Geometry check sheet. Reference: the model listing, model coordinates, mm. A direction names the side the tool comes from. Give positions to 0.01 mm unless a question says otherwise; leave off trailing zeros. Write each loop counter-clockwise with the first axis right and the second up, starting at its lowest first coordinate (ties: lowest second). Pieces come first, ordered by that corner, then holes.
(1) Cross-section at D-D (x = -6). Record the boundary of the cut face in (y, z).
(2) Mould release check, pull along Y, two halves, no side actions. Record for faces 4 (the flat face through (-10.447, 4.997, 0.071)), 5 (the flat face through (-19, -9.906, 0)), 6 (the flat face through (0, 20.32, 0)), 7 (the flat face through (-19, 0, 2.286)): +Y half, -Y half, draft (parallel to the pull), parting line (faces both ways), or undercut.
(3) Cross-section at C-C (y = 12). Record the boundary of the cut face in (x, z).
(4) Tool access check on faces 1 (the flat face through (-1, 11.232, 0)), 2 (the flat face through (-19, 9.906, 0)), 3 (the flat face through (-10.16, -17, 0)). Record the directions out of +Z, -Z, +X, -X, +Y, -Y that give a thin tool (end or side, any length) a straight path to the whole face; none if there is none.
(5) Cross-section at B-B (y = -8.5). Record the boundary of the cut face in (x, z), and give its area (3 significant figures).
(6) Depth check by flat-ended pin: P1, Ø1.3, axis at x = -18.5, z = -0.5, coming from the -Y side; P2, Ø1.3, axis at x = -19.5, z = 1, coming from the +Y side; P3, Ø12, axis at x = 0, y = 4, coming from the +Z side; P4, Ø1.3, axis at y = 19, z = 0, coming from the -X side. Enter the tip coordinate at first touch or a pass-through.
(7) Thickness scan on line 1 along X through (y, z) = (3.5, 1.25); line 2 along X through (y, z) = (-4.5, 0.5); line 3 along X through (y, z) = (8, -0.5). Record the ranges inside material, lowest first.
(8) Cross-section at A-A (x = 8). Record the boundary of the cut face in (y, z), and give its area (3 significant figures).
```python
from build123d import *

# Parameters (mm, degrees)
F0_W     = 35.56
F0_H     = 35.56
F1_DEPTH = 5.08
F2_W     = 19.812
F2_H     = 4.572
F3_DEPTH = 2.54
F4_W     = 19.812
F4_H     = 4.572
F5_DEPTH = 2.54
F6_W     = 20.32
F6_H     = 5.08
F7_DEPTH = 2.54
F8_W     = 20.32
F8_H     = 5.08
F9_DEPTH = 2.54


with BuildPart() as f1:
    # F0 (on Top) → F1 (new body, symmetric)
    with BuildSketch(Plane.XY):
        Rectangle(F0_W, F0_H)
        with BuildLine():
            Line((14.6379626736, 11.2322239583), (8.7401796875, -11.938))
            Line((8.7401796875, -11.938), (3.1466675347, -11.938))
            Line((3.1466675347, -11.938), (0.0076067708, 0.2328333333))
            add(Edge.make_bspline(
                [(0.0076067708, 0.2328333333), (-0.1648133681, 0.8819444444), (-0.5857213542, 2.9180234375)],
                knots=[0, 0, 0, 1, 1, 1], degree=2))
            add(Edge.make_bspline(
                [(-0.5857213542, 2.9180234375), (-1.0066293403, 4.9541024306), (-1.0674835069, 5.6539253472)],
                knots=[0, 0, 0, 1, 1, 1], degree=2))
            add(Edge.make_bspline(
                [(-1.0674835069, 5.6539253472), (-1.1638359375, 4.7968958333), (-1.5441744792, 2.9028098958)],
                knots=[0, 0, 0, 1, 1, 1], degree=2))
            add(Edge.make_bspline(
                [(-1.5441744792, 2.9028098958), (-1.9245130208, 1.0087239583), (-2.1324314236, 0.20240625)],
                knots=[0, 0, 0, 1, 1, 1], degree=2))
            Line((-2.1324314236, 0.20240625), (-5.2512074653, -11.938))
            Line((-5.2512074653, -11.938), (-10.8295060764, -11.938))
            Line((-10.8295060764, -11.938), (-16.7425026042, 11.2322239583))
            Line((-16.7425026042, 11.2322239583), (-11.9096675347, 11.2322239583))
            Line((-11.9096675347, 11.2322239583), (-8.9430269097, -1.4153003472))
            add(Edge.make_bspline(
                [(-8.9430269097, -1.4153003472), (-8.1671362847, -4.9194861111), (-7.8222960069, -7.4855034722)],
                knots=[0, 0, 0, 1, 1, 1], degree=2))
            add(Edge.make_bspline(
                [(-7.8222960069, -7.4855034722), (-7.7259435764, -6.5828333333), (-7.3836388889, -4.6887473958)],
                knots=[0, 0, 0, 1, 1, 1], degree=2))
            add(Edge.make_bspline(
                [(-7.3836388889, -4.6887473958), (-7.0413342014, -2.7946614583), (-6.7421345486, -1.7499982639)],
                knots=[0, 0, 0, 1, 1, 1], degree=2))
            Line((-6.7421345486, -1.7499982639), (-3.3647282986, 11.2322239583))
            Line((-3.3647282986, 11.2322239583), (1.2754019097, 11.2322239583))
            Line((1.2754019097, 11.2322239583), (4.6528081597, -1.7499982639))
            add(Edge.make_bspline(
                [(4.6528081597, -1.7499982639), (4.8759401042, -2.6171701389), (5.2081024306, -4.4098324653)],
                knots=[0, 0, 0, 1, 1, 1], degree=2))
            add(Edge.make_bspline(
                [(5.2081024306, -4.4098324653), (5.5402647569, -6.2024947917), (5.7126848958, -7.4855034722)],
                knots=[0, 0, 0, 1, 1, 1], degree=2))
            add(Edge.make_bspline(
                [(5.7126848958, -7.4855034722), (5.8698914931, -6.2481354167), (6.2198029514, -4.4022256944)],
                knots=[0, 0, 0, 1, 1, 1], degree=2))
            add(Edge.make_bspline(
                [(6.2198029514, -4.4022256944), (6.5697144097, -2.5563159722), (6.8537005208, -1.4153003472)],
                knots=[0, 0, 0, 1, 1, 1], degree=2))
            Line((6.8537005208, -1.4153003472), (9.8000564236, 11.2322239583))
            Line((9.8000564236, 11.2322239583), (14.6379626736, 11.2322239583))
        make_face(mode=Mode.SUBTRACT)
    extrude(amount=F1_DEPTH, both=True)

    # F2 (on face) → F3 (join)
    with BuildSketch(Plane(origin=(0, 17.78, 0), x_dir=(-1, 0, 0), z_dir=(0, 1, 0))):
        Rectangle(F2_W, F2_H)
    extrude(amount=F3_DEPTH)

    # F4 (on face) → F5 (join)
    with BuildSketch(Plane(origin=(-17.78, 0, 0), x_dir=(0, -1, 0), z_dir=(-1, 0, 0))):
        Rectangle(F4_W, F4_H)
    extrude(amount=F5_DEPTH)

    # F6 (on face) → F7 (cut)
    with BuildSketch(Plane.XZ.offset(17.78)):
        Rectangle(F6_W, F6_H)
    extrude(amount=-F7_DEPTH, mode=Mode.SUBTRACT)

    # F8 (on face) → F9 (cut)
    with BuildSketch(Plane.YZ.offset(17.78)):
        Rectangle(F8_W, F8_H)
    extrude(amount=-F9_DEPTH, mode=Mode.SUBTRACT)


solid = f1.part
```
Reply:
1. outline: (-17.78, -5.08) - (-11.94, -5.08) - (-11.94, 5.08) - (-17.78, 5.08) - (-17.78, 2.54) - (-15.24, 2.54) - (-15.24, -2.54) - (-17.78, -2.54) - close; (1.1, -5.08) - (17.78, -5.08) - (17.78, -2.29) - (20.32, -2.29) - (20.32, 2.29) - (17.78, 2.29) - (17.78, 5.08) - (1.1, 5.08) - close
2. face 4: undercut
2. face 5: -Y half
2. face 6: +Y half
2. face 7: draft
3. outline: (-17.78, -5.08) - (17.78, -5.08) - (17.78, 5.08) - (-17.78, 5.08) - close
4. face 1: +Z, -Z
4. face 2: +Z, -Z, -X, +Y
4. face 3: -Y
5. outline: (-20.32, -2.29) - (-17.78, -2.29) - (-17.78, -5.08) - (-11.71, -5.08) - (-11.71, 5.08) - (-17.78, 5.08) - (-17.78, 2.29) - (-20.32, 2.29) - close; (-4.37, -5.08) - (2.26, -5.08) - (2.26, 5.08) - (-4.37, 5.08) - close; (9.62, -5.08) - (17.78, -5.08) - (17.78, -2.54) - (15.24, -2.54) - (15.24, 2.54) - (17.78, 2.54) - (17.78, 5.08) - (9.62, 5.08) - close
5. area: 211 mm2
6. P1: stops at y = -9.91
6. P2: stops at y = 9.91
6. P3: stops at z = 5.08
6. P4: stops at x = -9.91
7. line 1: x = -20.32 to -14.77, -10.1 to -5.38, -1.43 to -0.7, 3.29 to 8, 12.67 to 15.24
7. line 2: x = -20.32 to -12.73, -8.31 to -7.35, -3.34 to 1.23, 5.22 to 6.2, 10.63 to 15.24
7. line 3: x = -20.32 to -15.92, -11.15 to -4.21, 2.12 to 9.05, 13.82 to 15.24
8. outline: (-17.78, -5.08) - (-11.94, -5.08) - (-11.94, 5.08) - (-17.78, 5.08) - (-17.78, 2.54) - (-15.24, 2.54) - (-15.24, -2.54) - (-17.78, -2.54) - close; (3.51, -5.08) - (17.78, -5.08) - (17.78, -2.29) - (20.32, -2.29) - (20.32, 2.29) - (17.78, 2.29) - (17.78, 5.08) - (3.51, 5.08) - close
8. area: 203 mm2
